Autodesk Inventor part; units mm, degrees
ref_plane "Start plane" through (0, 0, 21.2046) normal (0, 0, 1) x (1, 0, 0)
ref_plane "End plane" through (0, 0, 226.3838) normal (0, 0, 1) x (1, 0, 0)
ref_plane "Work Plane4" through (9, 112.687, 106.4266) normal (0, 0.727, 0.6866) x (1, 0, 0)
ref_plane "Start plane" through (0, 0, 21.2046) normal (0, 0, 1) x (1, 0, 0)
ref_plane "End plane" through (0, 0, 226.3838) normal (0, 0, 1) x (1, 0, 0)
sketch "Sketch" plane through (0, 0, 0) normal (0, 0, 1) x (1, 0, 0)
  line L0 (-15, -9) -> (-15, 9)
  line L1 (-9, 15) -> (9, 15)
  line L2 (15, 9) -> (15, -9)
  line L3 (9, -15) -> (-9, -15)
  arc A0 (-15, -9) -> (-9, -15) centre (-9, -9) ccw
  arc A1 (-9, 15) -> (-15, 9) centre (-9, 9) ccw
  arc A2 (15, 9) -> (9, 15) centre (9, 9) ccw
  arc A3 (9, -15) -> (15, -9) centre (9, -9) ccw
  arc A4 (-9, 12) -> (-12, 9) centre (-9, 9) ccw
  line L4 (-9, 12) -> (9, 12)
  arc A5 (12, 9) -> (9, 12) centre (9, 9) ccw
  line L5 (12, 9) -> (12, -9)
  arc A6 (9, -12) -> (12, -9) centre (9, -9) ccw
  line L6 (9, -12) -> (-9, -12)
  arc A7 (-12, -9) -> (-9, -12) centre (-9, -9) ccw
  line L7 (-12, -9) -> (-12, 9)
  line L8 (0, 22.7397) -> (0, -22.7397) construction
  line L9 (-22.7397, 0) -> (22.7397, 0) construction
  dimension "d7" = 6
  dimension "d10" = 30
  dimension "d11" = 30
  dimension "d12" = 3
  dimension "d15" = 15
  dimension "d16" = 15
extrude "Body" add sketch "Sketch" along normal up to surface (205.1793 mm away) from surface at 21.2046
sketch "Sketch3" plane through (0, 0, 0) normal (0, 0, 1) x (1, 0, 0)
  line L0 (0, 0) -> (10, 0)
ref_plane "Work Plane3" through (0, 0, 0) normal (0, -1, 0) x (1, 0, 0)
ref_plane "Work Plane4" through (9, 112.687, 106.4266) normal (0, 0.727, 0.6866) x (1, 0, 0)
split "Split1" plane through (9, 112.687, 106.4266) removes the side toward (0, 0.727, 0.6866)
ref_plane "Work Plane5" through (9, 10.2994, 236.6832) normal (0, -0.6866, 0.727) x (1, 0, 0)
split "Split2" plane through (9, 10.2994, 236.6832) removes the side toward (0, -0.6866, 0.727)
ref_plane "Work Plane6" through (9, -1028.8448, -951.0544) normal (0, 0.6866, -0.727) x (1, 0, 0)
split "Split3" plane through (9, -1028.8448, -951.0544) removes the side toward (0, 0.6866, -0.727)
ref_plane "Work Plane7" through (-9, 10.9052, 10.2994) normal (0, -0.727, -0.6866) x (1, 0, 0)
split "Split4" plane through (-9, 10.9052, 10.2994) removes the side toward (0, -0.727, -0.6866)
sketch "Sketch4" plane through (0, 0, 0) normal (0, -1, 0) x (1, 0, 0)
  line L0 (-2, 21.2046) -> (12, 21.2046)
  line L1 (-2, 226.3838) -> (12, 226.3838)
  dimension "d18" = 205.1793
equation "\"d7\" = G_IR"
equation "\"d10\" = G_H"
equation "\"d11\" = G_W"
equation "\"d12\" = G_T"
equation "\"d15\" = 0.5 * d10"
equation "\"d16\" = 0.5 * d11"
equation "\"d3\" = G_L"
equation "\"G_W\" = 30"
equation "\"G_H\" = 30"
equation "\"G_T\" = 3"
equation "\"G_IR\" = 6"
equation "\"G_L\" = d18"
equation "\"G_OFFSET_START\" = -21.20455"
equation "\"G_OFFSET_END\" = -21.20455"
equation "\"d13\" = -G_OFFSET_START"
equation "\"d14\" = G_OFFSET_END + B_L"
equation "\"B_L\" = 247.58837"
properties part number "DIN EN 10219-2 - 30 x 30 x 3  - 205.18" material "Steel, Mild"
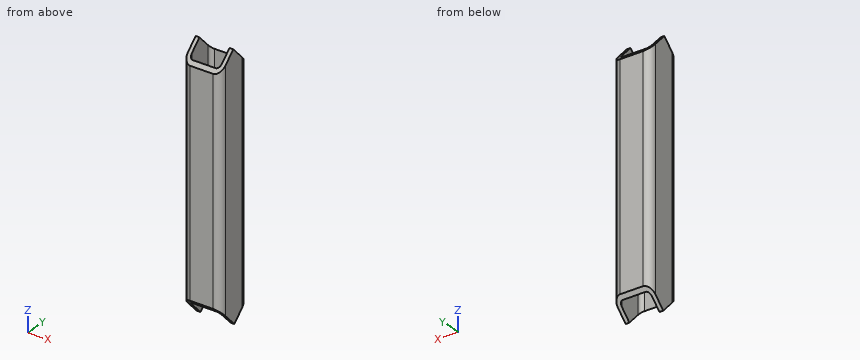
The listing builds one solid part. Answer for the finished solid, in the listing's coordinates (mm). Coordinates: 2 decimals unless noted, no trailing zeros. Order: outer loops, then holes, each group sorted by start corner. A loop starts at its lowest first (then second) coordinate and runs counter-clockwise, first axis right, second up.
Q1. A cutting plane is placed at B-B, the plane z = 41. Write down the section's boundary in (x, y), and give its area (3 significant figures).
Q2. Consider line 1 (Y direction, x = -8, z = 91); line 2 (Z direction, x = -11, y = -12). Determine where each line is inside the solid, lowest interval first.
Q3. A cutting plane is placed at C-C, the plane y = 7. Write down the section's boundary in (x, z), and give its area (3 significant figures).
Q4. A cutting plane is placed at A-A, the plane x = 4.75. Write down the section's boundary in (y, z).
Q5. Given P1, Ø10, axis at x = -3.5, y = 6.5, coming from the -Z side, flat-ended and moving along its own axis, determine where the tip first touches the part or whether it passes through.
Answers follow:
1. outline: (-15, -9) arc R6 ccw to (-9, -15) - (9, -15) arc R6 ccw to (15, -9) - (15, 9) arc R6 ccw to (9, 15) - (-9, 15) arc R6 ccw to (-15, 9) - close; hole (-12, -9) arc R3 ccw to (-9, -12) - (9, -12) arc R3 ccw to (12, -9) - (12, 9) arc R3 ccw to (9, 12) - (-9, 12) arc R3 ccw to (-12, 9) - close
1. area: 301 mm2
2. line 1: y = -15 to -12, 12 to 15
2. line 2: z = 34.55 to 215.62
3. outline: (-15, 27.23) - (-12, 27.23) - (-12, 218.33) - (-15, 218.33) - close; (12, 27.23) - (15, 27.23) - (15, 218.33) - (12, 218.33) - close
3. area: 1,150 mm2
4. outline: (-15, 37.73) - (-12, 34.55) - (-12, 215.62) - (-15, 212.79) - close; (12, 31.95) - (15, 34.78) - (15, 209.86) - (12, 213.04) - close
5. P1: passes through
